```python
from build123d import *

# Parameters (mm, degrees)
SKETCH1_W                = 32
SKETCH1_H                = 32
BOSS_EXTRUDE1_DEPTH      = 5
BOSS_EXTRUDE2_DEPTH      = 24
BOSS_EXTRUDE2_DEPTH_BACK = 21
SKETCH3_W                = 21.632810856
SKETCH3_H                = 9.374415515
CUT_EXTRUDE1_DEPTH       = 26
CUT_EXTRUDE3_DEPTH       = 3
BOSS_EXTRUDE3_REACH      = 38.453
BOSS_EXTRUDE4_REACH      = 39.779
CHAMFER2_SIZE            = 1
FILLET3_R                = 6
CHAMFER3_SIZE            = 1


with BuildPart() as part:
    # Sketch1 → Boss-Extrude1 (new body)
    with BuildSketch(Plane(origin=(0, 0, 0), x_dir=(1, 0, 0), z_dir=(0, 1, 0))):
        Rectangle(SKETCH1_W, SKETCH1_H)
    extrude(amount=BOSS_EXTRUDE1_DEPTH)

    # Sketch2 → Boss-Extrude2 (add, two sides: drawn at the far end of the back side and taken through both)
    with BuildSketch(Plane(origin=(0.604611907, 0.150768448, 0.604611907), x_dir=(0.7071067811865476, 0, -0.7071067811865476), z_dir=(0.6963642403200193, 0.17364817766692736, 0.6963642403200193)).offset(-BOSS_EXTRUDE2_DEPTH_BACK)):
        with BuildLine():
            Line((-4.469496616, 14), (-10.008100473, 14))
            Line((-10.008100473, 14), (-10.008100473, 2.732717447))
            Line((-10.008100473, 2.732717447), (9.991899527, 2.729904182))
            Line((9.991899527, 2.729904182), (9.991899527, 14))
            Line((9.991899527, 14), (4.469496616, 14))
            ThreePointArc((4.469496616, 14), (0, 8.42), (-4.469496616, 14))
        make_face()
    extrude(amount=BOSS_EXTRUDE2_DEPTH + BOSS_EXTRUDE2_DEPTH_BACK)

    # Sketch3 → Cut-Extrude1 (cut)
    with BuildSketch(Plane(origin=(-14.01903714, -3.495843283, -14.01903714), x_dir=(-0.6756735354111862, -0.16848866057223583, 0.7176885430348756), z_dir=(-0.6963642403200194, -0.17364817766692736, -0.6963642403200193))):
        with Locations((-1.423401453, 7.396880279)):
            Rectangle(SKETCH3_W, SKETCH3_H)
    extrude(amount=CUT_EXTRUDE1_DEPTH, mode=Mode.SUBTRACT)

    # Sketch4 → Cut-Extrude3 (cut)
    with BuildSketch(Plane(origin=(-14.01903714, -3.495843283, -14.01903714), x_dir=(-0.6756735354111862, -0.16848866057223583, 0.7176885430348756), z_dir=(-0.6963642403200194, -0.17364817766692736, -0.6963642403200193))):
        with BuildLine():
            Line((-2.760198528, 8.259804018), (-2.791216986, 8.402799894))
            Line((-2.791216986, 8.402799894), (-0.222019538, 8.960106488))
            Line((-0.222019538, 8.960106488), (-0.191719193, 8.722714198))
            ThreePointArc((-0.191719193, 8.722714198), (-1.330630481, 7.684897625), (-2.760198528, 8.259804018))
        make_face()
    extrude(amount=-CUT_EXTRUDE3_DEPTH, mode=Mode.SUBTRACT)

    # Boss-Extrude3: up to this face of the body (flat: up to its plane)
    boss_extrude3_end = Plane(part.part.faces().sort_by_distance((12.948102595, 6.004070548, 12.962810253))[0])
    # Sketch5 → Boss-Extrude3 (add, up to the picked face)
    with BuildSketch(Plane(origin=(0, 5, 0), x_dir=(1, 0, 0), z_dir=(0, 1, 0)), mode=Mode.PRIVATE) as boss_extrude3_sk1:
        Polygon((16, -1.869320176), (1.846408577, -16), (16, -16), align=None)
    boss_extrude3_tool1 = split(extrude(boss_extrude3_sk1.sketch, amount=BOSS_EXTRUDE3_REACH, mode=Mode.PRIVATE), bisect_by=boss_extrude3_end, keep=Keep.BOTH, mode=Mode.PRIVATE)
    add(boss_extrude3_tool1.solids().sort_by(Axis((11.282136, 5, 11.289773), (0, 1, 0)))[0])

    # Boss-Extrude4: up to this plane
    boss_extrude4_end = Plane(origin=(0, 0, 0), z_dir=(0, 1, 0))
    # Sketch6 → Boss-Extrude4 (add, up to the surface)
    with BuildSketch(Plane(origin=(-0.335099844, 2.689814891, -0.335643177), x_dir=(0.992445248624536, 0.12174417303820455, -0.015191603398808283), z_dir=(0.12268833882070036, -0.9848077432694324, 0.12288726668774345)), mode=Mode.PRIVATE) as boss_extrude4_sk1:
        Polygon((2.19811463, 16.495983278), (10.318063839, 24.741397108), (24.568201142, 10.708094048), (16.459446872, 2.474048136), (16.459446872, 16.714315992), align=None)
    boss_extrude4_tool1 = split(extrude(boss_extrude4_sk1.sketch, amount=BOSS_EXTRUDE4_REACH, mode=Mode.PRIVATE), bisect_by=boss_extrude4_end, keep=Keep.BOTH, mode=Mode.PRIVATE)
    add(boss_extrude4_tool1.solids().sort_by_distance((6.098904, 6.004719, 19.80612))[0])

    # Chamfer2
    # the kernel refuses this chamfer: 1 mm, written as the material it adds along each edge
    with BuildSketch(Plane(origin=(-13.061628157, 6.132633274, -13.069351365), x_dir=(-0.29592354594657705, 0.9534387650849755, 0.05817023455033625), z_dir=(0.6538395061159328, 0.2465782464577767, -0.7153272458224147))) as chamfer2_piece_1_section:
        Polygon((1.448815372, -CHAMFER2_SIZE), (1.448815372 - CHAMFER2_SIZE, 0), (1.448815372, 0), align=None)
    chamfer2_piece_1 = revolve(axis=Axis((-13.061628157, 6.132633274, -13.069351365), (0.6963642403200193, 0.17364817766692733, 0.6963642403200193)), revolution_arc=331.166542544, mode=Mode.PRIVATE)
    chamfer2_piece_1 = chamfer2_piece_1 - Plane(origin=(-13.810185227, 9.756782822, -13.810185227), x_dir=(0.6632365855153953, 0.21502352685856047, -0.7168557138861248), z_dir=(-0.6963642403200193, -0.1736481776669273, -0.6963642403200193)) * Cylinder(4.58, 6, mode=Mode.PRIVATE)
    add(chamfer2_piece_1)

    # Fillet3
    # the kernel refuses this fillet: 6 mm, written as the material it adds along each edge
    with BuildSketch(Plane(origin=(26.606601718, 5, 12.475921893), x_dir=(0, 1, 0), z_dir=(-0.7071067811865475, 0, -0.7071067811865476))) as fillet3_piece_1_section:
        with BuildLine():
            CenterArc((FILLET3_R, FILLET3_R), FILLET3_R, 180, 90)
            Line((0, FILLET3_R), (0, 0))
            Line((0, 0), (FILLET3_R, 0))
        make_face()
    fillet3_piece_1 = extrude(amount=55.271034943, mode=Mode.PRIVATE)
    fillet3_piece_1 = split(fillet3_piece_1, bisect_by=Plane(origin=(7.920941569, 6.446020655, -16), z_dir=(0, 0, 1)), keep=Keep.TOP, mode=Mode.PRIVATE)
    fillet3_piece_1 = split(fillet3_piece_1, bisect_by=Plane(origin=(16, 6.446020655, -7.920941569), z_dir=(-1, 0, 0)), keep=Keep.TOP, mode=Mode.PRIVATE)
    add(fillet3_piece_1)
    with BuildSketch(Plane(origin=(-26.606601718, 5, -12.453010295), x_dir=(0, 1, 0), z_dir=(0.7071067811865475, 0, 0.7071067811865476))) as fillet3_piece_2_section:
        with BuildLine():
            CenterArc((FILLET3_R, FILLET3_R), FILLET3_R, 180, 90)
            Line((0, FILLET3_R), (0, 0))
            Line((0, 0), (FILLET3_R, 0))
        make_face()
    fillet3_piece_2 = extrude(amount=55.238633049, mode=Mode.PRIVATE)
    fillet3_piece_2 = split(fillet3_piece_2, bisect_by=Plane(origin=(-16, 6.446146756, 7.932246434), z_dir=(1, 0, 0)), keep=Keep.TOP, mode=Mode.PRIVATE)
    fillet3_piece_2 = split(fillet3_piece_2, bisect_by=Plane(origin=(-7.932246434, 6.446146756, 16), z_dir=(0, 0, -1)), keep=Keep.TOP, mode=Mode.PRIVATE)
    add(fillet3_piece_2)

    # Chamfer3
    chamfer3_edges = [part.edges().sort_by_distance(p)[0] for p in [
        (16, 2.5, -16),
        (-16, 2.5, 16),
    ]]
    chamfer(chamfer3_edges, length=CHAMFER3_SIZE)


solid = part.part
```
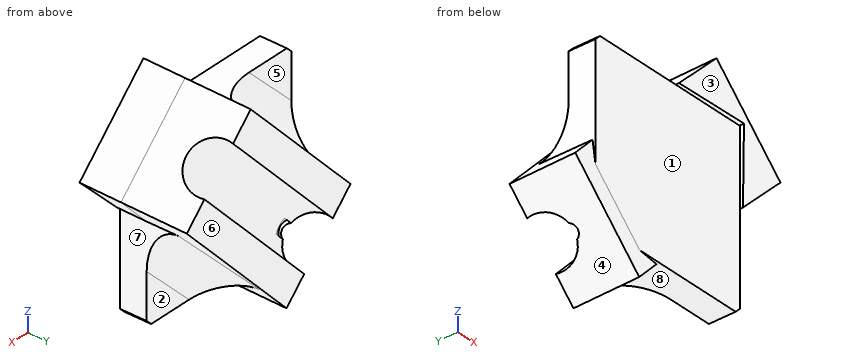
Here's how the part is built. I have some questions about the finished solid (model axes, mm). Face numbers are marked on the shaded views. A direction names the side the tool comes from. Round coordinates to 2 decimals unless told otherwise and drop trailing zeros. Write each loop counter-clockwise with the first axis right and the second up, starting at its lowest first coordinate (ties: lowest second). Pieces come first, ordered by that corner, then holes.
Q1. Will these pins go through, and if not, where does the flat tip stop? P1, Ø2, axis at x = 11, z = -2, coming from the -Y side; P2, Ø3.5, axis at x = -1.5, y = 6, coming from the +Z side; P3, Ø3, axis at x = -13, z = 10.5, coming from the +Y side.
Q2. If we section it at B-B on x = -19.5: Write out the boundary of the cut face in (y, z), plus the area to 3 significant figures.
Q3. Please list where these lines run through material, in increasing order: probe 1 along Y at (x, z) = (-13.5, 9); probe 2 along Z at (x, y) = (8, 0.75); probe 3 along X at (y, z) = (7.75, -8).
Q4. If we section it at A-A on y = 3: Write out the boundary of the cut face in (x, z).
Q5. Which directions (+Z, -Z, +X, -X, +Y, -Y) give clear straight access to the entire face, cutting with the end or side of a thin tool? Please do the marked faces 1, 2, 3, 4 and 5.
Q6. If we mould it in two halves opening along X, with no side actions, what happens to the marked faces 6, 7 and 8? For each: +X half, -X half, draft (parallel to the pull), parting line (faces both ways), or undercut.
Answer below:
1. P1: stops at y = 0
1. P2: stops at z = 16
1. P3: stops at y = 5.07
2. outline: (-0.81, -9.21) - (10.29, -11.98) - (11.12, -5.35) - (-0.32, -5.35) - close
2. area: 60.0 mm2
3. probe 1: y = 0 to 5
3. probe 2: z = -16 to 16, 16.62 to 22.15
3. probe 3: x = -22.15 to -13.16, -4.46 to 7.48
4. outline: (-21.91, -7.75) - (-7.76, -21.89) - (-1.87, -16) - (15, -16) - (16, -15) - (16, 16) - (-15, 16) - (-16, 15) - (-16, -1.85) - close; (2.1, 16.25) - (16.47, 16.47) - (16.25, 2.12) - (24.55, 10.42) - (10.4, 24.56) - close
5. face 1: +Z, +X, -Y
5. face 2: -Z, +X, +Y
5. face 3: +Z, -Z, +X, -X, -Y
5. face 4: -Z, -X, -Y
5. face 5: +Z, -X, +Y
6. face 6: -X half
6. face 7: undercut
6. face 8: draft
